Design review of the part built by this model. Coordinates are the model's own, in mm. A direction names the side the tool comes from. Give positions to 0.01 mm unless a question says otherwise; leave off trailing zeros. Write each loop counter-clockwise with the first axis right and the second up, starting at its lowest first coordinate (ties: lowest second). Pieces come first, ordered by that corner, then holes. Notation, with made-up numbers: (56, 53.5) - (87, 53.5) arc R26 cw to (87, 67.5) - close; hole circle Ø7 at (77.5, -20.5). An arc over 180 degrees is marked (long way). Use a Markdown table: item, result. Add a question column.
```python
from build123d import *

# Parameters (mm, degrees)
F0_W     = 150
F0_H     = 75
F1_DEPTH = 5
F3_DEPTH = 5.001
F5_DEPTH = 5.001
F6_W     = 25
F6_H     = 25
F7_DEPTH = 5.001
F8_R     = 10
F9_R     = 8


with BuildPart() as f1:
    # F0 (on Top) → F1 (new body)
    with BuildSketch(Plane.XY):
        with Locations((-34.16129, 0.826124)):
            Rectangle(F0_W, F0_H)
    extrude(amount=F1_DEPTH)

    # F2 (on face) → F3 (cut, through all)
    with BuildSketch(Plane.XY.offset(5)):
        with BuildLine():
            Line((-89.776412, 3.326124), (-89.776412, -36.673876))
            Line((-89.776412, -36.673876), (-69.776412, -36.673876))
            Line((-69.776412, -36.673876), (-69.776412, 3.326124))
            ThreePointArc((-69.776412, 3.326124), (-79.776412, 13.326124), (-89.776412, 3.326124))
        make_face()
    extrude(amount=-F3_DEPTH, mode=Mode.SUBTRACT)

    # F4 (on face) → F5 (cut, through all)
    with BuildSketch(Plane.XY.offset(5)):
        with BuildLine():
            Line((31.320997, -1.673876), (31.320997, 38.326124))
            Line((31.320997, 38.326124), (11.320997, 38.326124))
            Line((11.320997, 38.326124), (11.320997, -1.673876))
            ThreePointArc((11.320997, -1.673876), (21.320997, -11.673876), (31.320997, -1.673876))
        make_face()
    extrude(amount=-F5_DEPTH, mode=Mode.SUBTRACT)

    # F6 (on face) → F7 (cut, through all)
    with BuildSketch(Plane.XY.offset(5)):
        with Locations((-24.330012, 4.958801)):
            Rectangle(F6_W, F6_H)
    extrude(amount=-F7_DEPTH, mode=Mode.SUBTRACT)

    # F8
    f8_edges = [f1.edges().sort_by_distance(p)[0] for p in [
        (-36.830012, -7.541199, 2.5),
        (-11.830012, -7.541199, 2.5),
        (-11.830012, 17.458801, 2.5),
        (-36.830012, 17.458801, 2.5),
    ]]
    fillet(f8_edges, radius=F8_R)

    # F9
    f9_edges = [f1.edges().sort_by_distance(p)[0] for p in [
        (40.83871, 38.326124, 2.5),
        (-109.16129, -36.673876, 2.5),
        (40.83871, -36.673876, 2.5),
        (-109.16129, 38.326124, 2.5),
    ]]
    fillet(f9_edges, radius=F9_R)


solid = f1.part
```
(1) Add section C-C (y = 1). State the section outline as (x, z) points, and give its area (3 significant figures).
(2) Tool access review of faces 1 (the face through (38.433, 36.045, 2.535)), 2 (the face through (-69.776, -17, 3)), 3 (the face through (-33.82, -4.69, 2.46)), 4 (the face through (11.321, 19, 3)), 5 (the face through (-106.9, 35.9, 2.5)): name each direction out of +Z, -Z, +X, -X, +Y, -Y from which nothing blocks a thin tool from reaching the whole face with its end or side.
(3) Mouldability with a two-part tool opening along Y and no side actions: class faces 6 (the face through (-79.557, 13.324, 2.535)), 7 (the face through (-35, -7, 5)), 8 (the face through (-24, -7.541, 3)) as +Y half, -Y half, draft (parallel to the pull), parting line (faces both ways), or undercut.
(4) Add section D-D (y = 15.5). State the section outline as (x, z) points.
(5) Insertion check: pin 1 (5 mm diameter, centred on x = -60, y = 13.5, fed in from -Z); pin 2 (1.5 mm diameter, centred on x = -76, z = 1, fed in from -Y). Each pin has a flat end and moves straight along its axis. Give the tip position at first contact, or say it passes through.
(6) Add section A-A (z = 0.8). State the section outline as (x, y) points.
(7) Add section B-B (y = -21). State the section outline as (x, z) points, and give its area (3 significant figures).
(8) For line 1 along X through (y, z) = (4, 4.15); line 2 along Y through (x, z) = (-24, 4.15); line 3 along X through (y, z) = (20, 0.8), list the stretches that pass through material, from the lowest coordinate up.
Answers follow:
| question | item | result |
|---|---|---|
| 1 | outline | (-109.16, 0) - (-89.78, 0) - (-89.78, 5) - (-109.16, 5) - close; (-69.78, 0) - (-36.72, 0) - (-36.72, 5) - (-69.78, 5) - close; (-11.94, 0) - (11.32, 0) - (11.32, 5) - (-11.94, 5) - close; (31.32, 0) - (40.84, 0) - (40.84, 5) - (31.32, 5) - close |
| 1 | area | 426 mm^2 |
| 2 | face 1 | +Z, -Z, +X, +Y |
| 2 | face 2 | +Z, -Z, -Y |
| 2 | face 3 | +Z, -Z |
| 2 | face 4 | +Z, -Z, +Y |
| 2 | face 5 | +Z, -Z, -X, +Y |
| 3 | face 6 | -Y half |
| 3 | face 7 | draft |
| 3 | face 8 | undercut |
| 4 | outline | (-109.16, 0) - (-32.77, 0) - (-32.77, 5) - (-109.16, 5) - close; (-15.89, 0) - (11.32, 0) - (11.32, 5) - (-15.89, 5) - close; (31.32, 0) - (40.84, 0) - (40.84, 5) - (31.32, 5) - close |
| 5 | pin 1 | z = 0 |
| 5 | pin 2 | y = 12.24 |
| 6 | outline | (-109.16, -28.67) arc R8 ccw to (-101.16, -36.67) - (-89.78, -36.67) - (-89.78, 3.33) arc R10 cw to (-69.78, 3.33) - (-69.78, -36.67) - (32.84, -36.67) arc R8 ccw to (40.84, -28.67) - (40.84, 30.33) arc R8 ccw to (32.84, 38.33) - (31.32, 38.33) - (31.32, -1.67) arc R10 cw to (11.32, -1.67) - (11.32, 38.33) - (-101.16, 38.33) arc R8 ccw to (-109.16, 30.33) - close; hole (-36.83, 2.46) arc R10 ccw to (-26.83, -7.54) - (-21.83, -7.54) arc R10 ccw to (-11.83, 2.46) - (-11.83, 7.46) arc R10 ccw to (-21.83, 17.46) - (-26.83, 17.46) arc R10 ccw to (-36.83, 7.46) - close |
| 7 | outline | (-109.16, 0) - (-89.78, 0) - (-89.78, 5) - (-109.16, 5) - close; (-69.78, 0) - (40.84, 0) - (40.84, 5) - (-69.78, 5) - close |
| 7 | area | 650 mm^2 |
| 8 | line 1 | -109.16 to -89.75, -69.8 to -36.83, -11.83 to 11.32, 31.32 to 40.84 |
| 8 | line 2 | -36.67 to -7.54, 17.46 to 38.33 |
| 8 | line 3 | -109.16 to 11.32, 31.32 to 40.84 |
